Check sheet for the modelled part. Datum: model origin and axes. Units: mm. A direction names the side the tool comes from. Coordinates: 2 decimals unless noted, no trailing zeros. Loops run counter-clockwise (first coordinate to the right, second up) from the corner with the lowest first, then second, coordinate; pieces in that order, holes last. Notation, with made-up numbers: (19, -9) - (53, -9) arc R17 cw to (53, 22) - close; hole circle Ø7 at (66.5, 89.25). An arc over 180 degrees is marked (long way). Write each question's results on one line, items separated by ' | '. Start each with the question number.
1. Thickness scan on line 1 (Z direction, x = -113, y = -20); line 2 (Y direction, x = -205, z = 8); line 3 (Z direction, x = -17, y = -25). Record the ranges inside material, lowest first. Write a range as [from, to].
2. Cross-section at B-B (y = -11.5). Record the cut outline in (x, z), and give its area (3 significant figures).
3. Cross-section at C-C (z = 6.5). Record the cut outline in (x, y).
4. Cross-section at D-D (x = -224). Record the cut outline in (y, z), and give its area (3 significant figures).
5. Cross-section at A-A (x = -161.5). Record the cut outline in (y, z).
6. Tool access check on faces 1 (the face through (-121, -24, 15)), 2 (the face through (-121, -27, 13)). Record the directions out of +Z, -Z, +X, -X, +Y, -Y that give a thin tool (end or side, any length) a straight path to the whole face; none if there is none.
7. Gauge pin test, flat ends, axial feed: P1, Ø2.5, axis at y = -25, z = 18.5, coming from the -X side; P2, Ø1, axis at x = -83, z = 17, coming from the +Y side; P3, Ø3.5, axis at y = -25, z = 19, coming from the +X side; P4, Ø6, axis at x = -104.5, y = -13, coming from the -Z side. Record the tip position at first contact, or that the pin passes through.
```python
from build123d import *

# Parameters (mm, degrees)
SKETCH2_W           = 239
SKETCH2_H           = 27
BOSS_EXTRUDE1_DEPTH = 3
SKETCH3_W           = 239
SKETCH3_H           = 3
BOSS_EXTRUDE2_DEPTH = 12
BOSS_EXTRUDE4_DEPTH = 3


with BuildPart() as part:
    # Sketch2 → Boss-Extrude1 (new body)
    with BuildSketch(Plane.XY):
        with Locations((-119.5, -13.5)):
            Rectangle(SKETCH2_W, SKETCH2_H)
    extrude(amount=BOSS_EXTRUDE1_DEPTH)

    # Sketch3 → Boss-Extrude2 (add)
    with BuildSketch(Plane.XY.offset(3)):
        with Locations((-119.5, -25.5)):
            Rectangle(SKETCH3_W, SKETCH3_H)
    extrude(amount=BOSS_EXTRUDE2_DEPTH)

    # Sketch4 → Boss-Extrude4 (add)
    with BuildSketch(Plane(origin=(0, -24, 0), x_dir=(1, 0, 0), z_dir=(0, 1, 0))):
        with BuildLine():
            Line((-203, -15), (-36, -15))
            Line((-36, -15), (-36, -21))
            ThreePointArc((-36, -21), (-37.757359313, -25.242640687), (-42, -27))
            Line((-42, -27), (-197, -27))
            ThreePointArc((-197, -27), (-201.242640687, -25.242640687), (-203, -21))
            Line((-203, -21), (-203, -15))
        make_face()
    extrude(amount=-BOSS_EXTRUDE4_DEPTH)


solid = part.part
```
Established:
1) line 1: [0, 3] | line 2: [-27, -24] | line 3: [0, 15]
2) outline: (-239, 0) - (0, 0) - (0, 3) - (-239, 3) - close | area: 717 mm^2
3) outline: (-239, -27) - (0, -27) - (0, -24) - (-239, -24) - close
4) outline: (-27, 0) - (0, 0) - (0, 3) - (-24, 3) - (-24, 15) - (-27, 15) - close | area: 117 mm^2
5) outline: (-27, 0) - (0, 0) - (0, 3) - (-24, 3) - (-24, 27) - (-27, 27) - close
6) face 1: +Z, +X, -X, +Y | face 2: +Z, -Z, +X, -X, -Y
7) P1: x = -203 | P2: y = -24 | P3: x = -36 | P4: z = 0
